Geometry: final body of the model. Coordinates: model frame, mm. A direction names the side the tool comes from. Give positions to 0.01 mm unless a question says otherwise; leave off trailing zeros. Order: outer loops, then holes, each group sorted by start corner. A loop starts at its lowest first (then second) coordinate and runs counter-clockwise, first axis right, second up. Notation, with made-up numbers: (69.25, -38) - (127.25, -38) arc R30 ccw to (127.25, -15) - close; hole circle Ø3 at (49.5, -19). An arc over 180 degrees is marked (long way). One line per item, written item: value.
```python
from build123d import *

# Parameters (mm, degrees)
SKETCH1_R           = 12.5
BOSS_EXTRUDE1_DEPTH = 2
SKETCH2_R           = 5
BOSS_EXTRUDE2_DEPTH = 5.5
SKETCH3_R           = 2.75
CUT_EXTRUDE1_DEPTH  = 3
CUT_EXTRUDE2_REACH  = 21.203
SKETCH4_R           = 1
SKETCH5_R           = 3
CUT_EXTRUDE3_DEPTH  = 3
CUT_EXTRUDE4_REACH  = 20.241
SKETCH6_R           = 1.5


with BuildPart() as part:
    # Sketch1 → Boss-Extrude1 (new body)
    with BuildSketch(Plane(origin=(0, 0, 0), x_dir=(1, 0, 0), z_dir=(0, 1, 0))):
        with Locations(Location((0, 0, 0), (0, 0, 270))):
            Circle(SKETCH1_R)
    extrude(amount=BOSS_EXTRUDE1_DEPTH)

    # Sketch2 → Boss-Extrude2 (add)
    with BuildSketch(Plane.XZ):
        with Locations(Location((0, 0, 0), (0, 0, 90))):
            Circle(SKETCH2_R)
    extrude(amount=BOSS_EXTRUDE2_DEPTH)

    # Sketch3 → Cut-Extrude1 (cut)
    with BuildSketch(Plane.XZ.offset(5.5)):
        with Locations(Location((0, 0, 0), (0, 0, 270))):
            Circle(SKETCH3_R)
    extrude(amount=-CUT_EXTRUDE1_DEPTH, mode=Mode.SUBTRACT)

    # Sketch4 → Cut-Extrude2 (cut, up to next)
    with BuildSketch(Plane(origin=(0, 2, 0), x_dir=(1, 0, 0), z_dir=(0, 1, 0)), mode=Mode.PRIVATE) as cut_extrude2_sk1:
        with Locations(Location((0, 8.5, 0), (0, 0, 270))):
            Circle(SKETCH4_R)
    cut_extrude2_tool1 = extrude(cut_extrude2_sk1.sketch, amount=-CUT_EXTRUDE2_REACH, mode=Mode.PRIVATE) & part.part
    # Sketch4 → Cut-Extrude2 (cut, up to next)
    with BuildSketch(Plane(origin=(0, 2, 0), x_dir=(1, 0, 0), z_dir=(0, 1, 0)), mode=Mode.PRIVATE) as cut_extrude2_sk2:
        with Locations(Location((0, -8.5, 0), (0, 0, 270))):
            Circle(SKETCH4_R)
    cut_extrude2_tool2 = extrude(cut_extrude2_sk2.sketch, amount=-CUT_EXTRUDE2_REACH, mode=Mode.PRIVATE) & part.part
    add(cut_extrude2_tool1.solids().sort_by_distance((0, 2, -8.5))[0], mode=Mode.SUBTRACT)
    add(cut_extrude2_tool2.solids().sort_by_distance((0, 2, 8.5))[0], mode=Mode.SUBTRACT)

    # Sketch5 → Cut-Extrude3 (cut)
    with BuildSketch(Plane(origin=(0, 2, 0), x_dir=(1, 0, 0), z_dir=(0, 1, 0))):
        with Locations(Location((0, 0, 0), (0, 0, 270))):
            Circle(SKETCH5_R)
    extrude(amount=-CUT_EXTRUDE3_DEPTH, mode=Mode.SUBTRACT)

    # Sketch6 → Cut-Extrude4 (cut, up to next)
    with BuildSketch(Plane(origin=(0, -1, 0), x_dir=(1, 0, 0), z_dir=(0, 1, 0)), mode=Mode.PRIVATE) as cut_extrude4_sk1:
        with Locations(Location((0, 0, 0), (0, 0, 270))):
            Circle(SKETCH6_R)
    cut_extrude4_tool1 = extrude(cut_extrude4_sk1.sketch, amount=-CUT_EXTRUDE4_REACH, mode=Mode.PRIVATE) & part.part
    add(cut_extrude4_tool1.solids().sort_by_distance((0, -1, 0))[0], mode=Mode.SUBTRACT)


solid = part.part
```
1) Section B-B, the plane z = 0. Return loops of the section in (x, y), then the cut area to 3 significant figures.
Answers below:
outline: (-12.5, 0) - (-5, 0) - (-5, -5.5) - (-2.75, -5.5) - (-2.75, -2.5) - (-1.5, -2.5) - (-1.5, -1) - (-3, -1) - (-3, 2) - (-12.5, 2) - close; (1.5, -2.5) - (2.75, -2.5) - (2.75, -5.5) - (5, -5.5) - (5, 0) - (12.5, 0) - (12.5, 2) - (3, 2) - (3, -1) - (1.5, -1) - close
area: 66.0 mm^2
2) Material intervals for line 1 along X through (y, z) = (0.35, 0); line 2 along X through (y, z) = (-3.2, 0); line 3 along Y through (x, z) = (1.5, 10.75), sorted ascending.
Answers below:
line 1: -12.5 to -3, 3 to 12.5
line 2: -5 to -2.75, 2.75 to 5
line 3: 0 to 2
3) Section D-D, the plane y = 0.5. Return loops of the section in (x, z).
Answers below:
outline: circle Ø25 at (0, 0); hole circle Ø6 at (0, 0); hole circle Ø2 at (0, -8.5); hole circle Ø2 at (0, 8.5)
4) Section C-C, the plane y = -3.5. Return loops of the section in (x, z).
Answers below:
outline: circle Ø10 at (0, 0); hole circle Ø5.5 at (0, 0)
5) Set-up query: faces 1 (the face through (0.9, 0.52, 2.86)), 2 (the face through (3.755, 0.986, 11.923)), 3 (the face through (-2.685, -4.021, 0.596)). Return all of +Z, -Z, +X, -X, +Y, -Y with unobstructed straight access to the full face (end or side cutting, diameter ignored); none if empty.
Answers below:
face 1: +Y
face 2: +Y, -Y
face 3: -Y
6) Mould query, pull axis Z, two halves, no side actions, for faces 4 (the face through (2.2, -5.5, 2.2)), 5 (the face through (4.88, -2.71, -1.08)), 6 (the face through (-1.3, -1, 1.3)). Classes: released by +Z, released by -Z, zero draft, split by the parting line, or undercut.
Answers below:
face 4: zero draft
face 5: split by the parting line
face 6: undercut
7) Section A-A, the plane x = 0. Return loops of the section in (y, z).
Answers below:
outline: (-5.5, -5) - (0, -5) - (0, -7.5) - (2, -7.5) - (2, -3) - (-1, -3) - (-1, -1.5) - (-2.5, -1.5) - (-2.5, -2.75) - (-5.5, -2.75) - close; (-5.5, 2.75) - (-2.5, 2.75) - (-2.5, 1.5) - (-1, 1.5) - (-1, 3) - (2, 3) - (2, 7.5) - (0, 7.5) - (0, 5) - (-5.5, 5) - close; (0, -12.5) - (2, -12.5) - (2, -9.5) - (0, -9.5) - close; (0, 9.5) - (2, 9.5) - (2, 12.5) - (0, 12.5) - close
8) First-contact query: pin 1 (4 mm diameter, centred on x = 0, z = 0, fed in from -Y); pin 2 (3 mm diameter, centred on x = -9.5, y = 0.5, fed in from -Z); pin 3 (4.5 mm diameter, centred on x = 0, z = 0, fed in from +Y). Flat tips, straight axial feed; report the tip coordinate or a pass-through.
Answers below:
pin 1: y = -2.5
pin 2: z = -9.6
pin 3: y = -1
